Here's the drawing with two shaded views (mm, measured from the low corner). I have some questions. Round coordinates to 2 decimals unless told otherwise and drop trailing zeros. Order: outer loops, then holes, each group sorted by start corner. A loop starts at its lowest first (then second) coordinate and runs counter-clockwise, first axis right, second up.
Q1. If we section it at A-A (x = 95.25): Please give me the cut outline in (y, z), plus the area to 3 significant figures.
Q2. Will this pin go through, and if not, where does the flat tip stop? P1, Ø3, axis at x = 95.25, z = 151.6, coming from the -Y side.
Q3. If I drill on line 1 (Z direction, x = 95.25, y = 10); line 2 (X direction, y = 8.5, z = 151.6); line 3 (X direction, y = 10, z = 152.5), over which ranges is the centre line in solid material (lowest first)?
Q4. If we section it at B-B (z = 151.6): Please give me the cut outline in (x, y), plus the area to 3 significant figures.
Q5. If we section it at C-C (y = 9.5): Count the separate pieces of the cut face and the enclosed holes in it, plus the area to 3 significant figures.
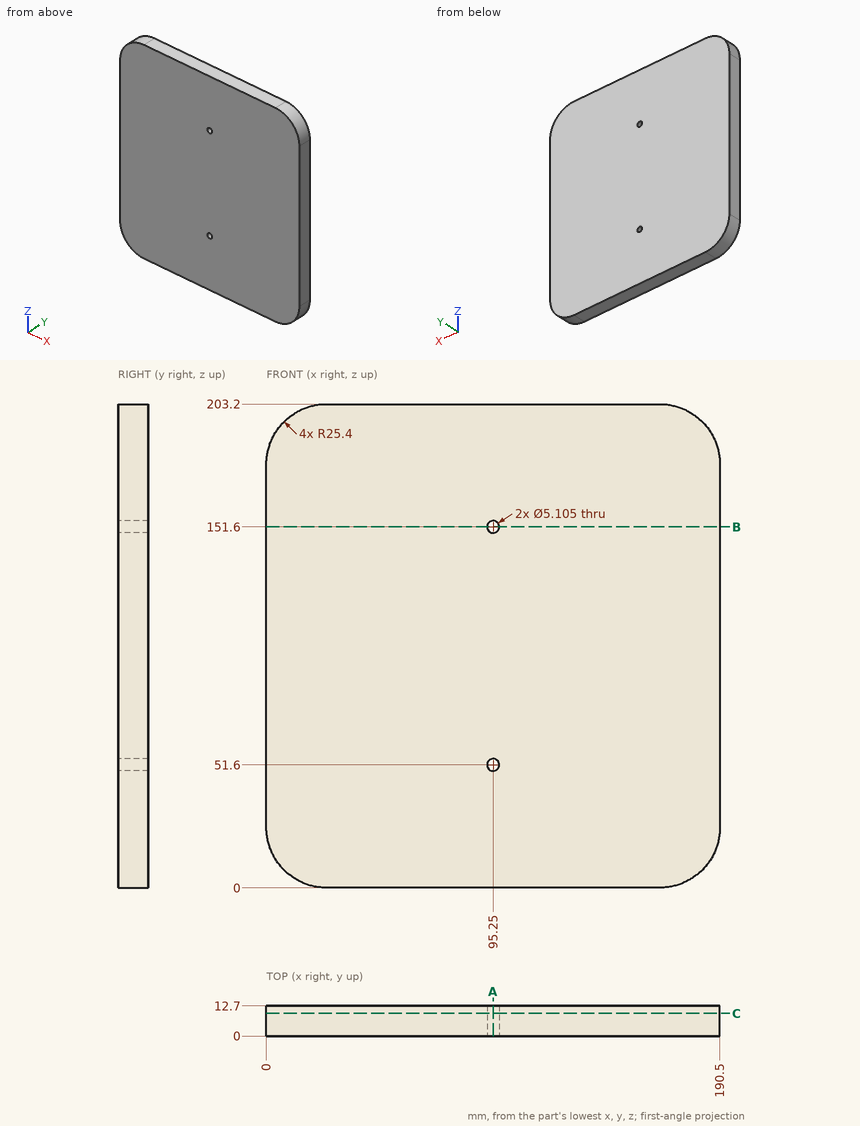
Solution:
1. outline: (0, 0) - (12.7, 0) - (12.7, 49.05) - (0, 49.05) - close; (0, 54.15) - (12.7, 54.15) - (12.7, 149.05) - (0, 149.05) - close; (0, 154.15) - (12.7, 154.15) - (12.7, 203.2) - (0, 203.2) - close
1. area: 2,450 mm2
2. P1: passes through
3. line 1: z = 0 to 49.05, 54.15 to 149.05, 154.15 to 203.2
3. line 2: x = 0 to 92.7, 97.8 to 190.5
3. line 3: x = 0 to 92.86, 97.64 to 190.5
4. outline: (0, 0) - (92.7, 0) - (92.7, 12.7) - (0, 12.7) - close; (97.8, 0) - (190.5, 0) - (190.5, 12.7) - (97.8, 12.7) - close
4. area: 2,350 mm2
5. separate pieces: 1
5. enclosed holes: 2
5. area: 38,100 mm2
